from build123d import *

# Parameters (mm, degrees)
SKETCH1_W                   = 50.8
SKETCH1_H                   = 25.4
BOSS_EXTRUDE1_DEPTH         = 3.175
F_1_4_0_25_DIAMETER_HOLE1_D = 6.35
SKETCH4_W                   = 50.8
SKETCH4_H                   = 6.35
SKETCH4_H_2                 = 4
BOSS_EXTRUDE2_DEPTH         = 19.05
CUT_EXTRUDE1_DEPTH          = 6.35
F_1_4_0_25_DIAMETER_HOLE2_D = 6.35
FILLET1_R                   = 18
CHAMFER1_SIZE               = 7


with BuildPart() as part:
    # Sketch1 → Boss-Extrude1 (new body)
    with BuildSketch(Plane.XY):
        Rectangle(SKETCH1_W, SKETCH1_H)
    extrude(amount=BOSS_EXTRUDE1_DEPTH)

    # 1/4 (0.25) Diameter Hole1 (through all)
    with Locations(Plane(origin=(0, 0, 0), x_dir=(-1, 0, 0), z_dir=(0, 0, -1))):
        with Locations((-12.7, 0), (12.7, 0)):
            Hole(F_1_4_0_25_DIAMETER_HOLE1_D / 2)

    # Sketch4 → Boss-Extrude2 (add)
    with BuildSketch(Plane(origin=(0, 0, 0), x_dir=(-1, 0, 0), z_dir=(0, 0, -1))):
        with Locations((0, -15.875)):
            Rectangle(SKETCH4_W, SKETCH4_H)
        with Locations((0, -10.7)):
            Rectangle(SKETCH4_W, SKETCH4_H_2)
    extrude(amount=BOSS_EXTRUDE2_DEPTH)

    # Sketch5 → Cut-Extrude1 (cut)
    with BuildSketch(Plane.XZ.offset(19.05)):
        Polygon((-3.299556788, -15.24), (3.299556788, -15.24), (6.599113577, -9.525), (3.299556788, -3.81), (-3.299556788, -3.81), (-6.599113577, -9.525), align=None)
    extrude(amount=-CUT_EXTRUDE1_DEPTH, mode=Mode.SUBTRACT)

    # 1/4 (0.25) Diameter Hole2 (through all)
    with Locations(Plane(origin=(0, -19.05, 0), x_dir=(-1, 0, 0), z_dir=(0, -1, 0))):
        with Locations((0, 9.525)):
            Hole(F_1_4_0_25_DIAMETER_HOLE2_D / 2)

    # Fillet1
    fillet1_edges = [part.edges().sort_by_distance(p)[0] for p in [
        (-25.4, -13.875, -19.05),
        (25.4, -13.875, -19.05),
    ]]
    fillet(fillet1_edges, radius=FILLET1_R)

    # Chamfer1
    # the kernel refuses this chamfer: 7 mm, written as the material it adds along each edge
    with BuildSketch(Plane(origin=(25.4, -12.7, 0), x_dir=(0, -0.9996219169112968, -0.02749587661058637), z_dir=(-1, 0, 0))) as chamfer1_piece_1_section:
        Polygon((CHAMFER1_SIZE * 0.999621916911, CHAMFER1_SIZE * 0.0274958766106), (-CHAMFER1_SIZE * 0.0274958766106, CHAMFER1_SIZE * 0.999621916911), (0, 0), align=None)
    chamfer1_piece_1 = extrude(amount=50.8, mode=Mode.PRIVATE)
    chamfer1_piece_1 = split(chamfer1_piece_1, bisect_by=Plane(origin=(0, -19.05, 1.366790838), z_dir=(0, 1, 0)), keep=Keep.TOP, mode=Mode.PRIVATE)
    chamfer1_piece_1 = split(chamfer1_piece_1, bisect_by=Plane(origin=(0, -15.42419562, 3.175), z_dir=(0, 0, -1)), keep=Keep.TOP, mode=Mode.PRIVATE)
    add(chamfer1_piece_1)


solid = part.part
Verification items for the finished model (mm, model axes). A direction names the side the tool comes from. Round coordinates to 2 decimals unless told otherwise and drop trailing zeros. Loops run counter-clockwise (first coordinate to the right, second up) from the corner with the lowest first, then second, coordinate; pieces in that order, holes last. Notation, with made-up numbers: M 35,87.25 L 55,87.25 A23 cw 55,95.25 Z; hole C 66.5,29 d8. An arc over 180 degrees is marked long. Write each question's results on one line, items separated by ' | '.
1) Section check C-C on z = 1.75. Record the boundary of the cut face in (x, y) (3 decimals), then the cut area to 3 significant figures.
Checks:
outline: M -25.4,-17.95 L 25.4,-17.95 L 25.4,12.7 L -25.4,12.7 Z; hole C -12.7,0 d6.35; hole C 12.7,0 d6.35 | area: 1,490 mm2
2) Mould release check, pull along Y, two halves, no side actions. Record for faces 1 (the flat face through (-4.926, -15.919, -6.627)), 2 (the cylindrical face through (-9.67, 0.95, 1.61)), 3 (the flat face through (0.4, -17.8, 1.9)), 4 (the cylindrical face through (9.53, 0.14, 1.61)): released by +Y, released by -Y, zero draft, split by the parting line, or undercut.
Checks:
face 1: zero draft | face 2: undercut | face 3: released by -Y | face 4: undercut
3) Gauge pin test, flat ends, axial feed: P1, Ø6, axis at x = -10.5, z = -12, coming from the +Y side; P2, Ø5.5, axis at x = 0.5, z = -9.5, coming from the -Y side; P3, Ø4, axis at y = -9, z = -16.5, coming from the +X side. Record the tip position at first contact, or that the pin passes through.
Checks:
P1: stops at y = -8.7 | P2: stops at y = -12.7 | P3: stops at x = 19.36
4) Section check D-D on y = -13.5. Record the boundary of the cut face in (x, z) (3 decimals).
Checks:
outline: M -25.4,-1.05 A18 ccw -7.4,-19.05 L 7.4,-19.05 A18 ccw 25.4,-1.05 L 25.4,3.175 L -25.4,3.175 Z; hole M -6.599,-9.525 L -3.3,-15.24 L 3.3,-15.24 L 6.599,-9.525 L 3.3,-3.81 L -3.3,-3.81 Z
5) Section check B-B on y = 0. Record the boundary of the cut face in (x, z) (3 decimals).
Checks:
outline: M -25.4,0 L -15.875,0 L -15.875,3.175 L -25.4,3.175 Z; M -9.525,0 L 9.525,0 L 9.525,3.175 L -9.525,3.175 Z; M 15.875,0 L 25.4,0 L 25.4,3.175 L 15.875,3.175 Z
6) Scan lines: L1, parallel to Z at x = 0, y = -11.25 (3 decimals); L2, parallel to Z at x = 3, y = -15 (3 decimals); L3, parallel to X at y = -0.5, z = 0.25. Record each from-to range of solid material in increasing order. Write a range as from..to.
Checks:
L1: z = -19.05..-12.7, -6.35..3.175 | L2: z = -19.05..-15.24, -3.81..3.175 | L3: x = -25.4..-15.84, -9.56..9.56, 15.84..25.4
7) Access from +Z, -Z, +X, -X, +Y, -Y to the whole of each face (thin tool, end or side, straight path). Record for faces 5 (the flat face through (25.4, -3, 1)), 6 (the flat face through (0, -8.7, -5)), 7 (the flat face through (4.926, -15.919, -12.423)).
Checks:
face 5: +Z, -Z, +X, +Y, -Y | face 6: -Z, +X, -X, +Y | face 7: -Y
8) Section check A-A on x = 0. Record the boundary of the cut face in (y, z) (3 decimals), then the cut area to 3 significant figures.
Checks:
outline: M -19.05,-19.05 L -8.7,-19.05 L -8.7,-12.7 L -12.7,-12.7 L -12.7,-15.24 L -19.05,-15.24 Z; M -19.05,-3.81 L -12.7,-3.81 L -12.7,-6.35 L -8.7,-6.35 L -8.7,0 L 12.7,0 L 12.7,3.175 L -16.525,3.175 L -19.05,0.65 Z | area: 197 mm2
